Design review of the part built by this model. Coordinates are the model's own, in mm. A direction names the side the tool comes from. Give positions to 0.01 mm unless a question says otherwise; leave off trailing zeros. Loops run counter-clockwise (first coordinate to the right, second up) from the corner with the lowest first, then second, coordinate; pieces in that order, holes last. Notation, with made-up numbers: M 7.25,-28.75 L 37.25,-28.75 A17 cw 37.25,-0.75 Z; hole C -10.5,86.5 d3. An arc over 180 degrees is marked long. Answer as CSV lines item,"result".
```python
from build123d import *

# Parameters (mm, degrees)
F0_W     = 60
F0_H     = 200
F1_DEPTH = 10
F2_W     = 30
F2_H     = 20
F3_DEPTH = 30
F4_W     = 50
F4_H     = 152
F5_DEPTH = 8
F6_R     = 12.472601
F7_DEPTH = 60.001


with BuildPart() as f1:
    # F0 (on Top) → F1 (new body)
    with BuildSketch(Plane.XY):
        Rectangle(F0_W, F0_H)
    extrude(amount=F1_DEPTH)

    # F2 (on Right) → F3 (join, symmetric)
    with BuildSketch(Plane.YZ):
        with Locations((-85, -10)):
            Rectangle(F2_W, F2_H)
        with Locations((85, -10)):
            Rectangle(F2_W, F2_H)
    extrude(amount=F3_DEPTH, both=True)

    # F4 (on face) → F5 (join)
    with BuildSketch(Plane.XY.offset(10)):
        Rectangle(F4_W, F4_H)
    extrude(amount=F5_DEPTH)

    # F6 (on face) → F7 (cut, through all)
    with BuildSketch(Plane.YZ.offset(30)):
        with Locations((-85, -5)):
            Circle(F6_R)
        with Locations((85, -5)):
            Circle(F6_R)
    extrude(amount=-F7_DEPTH, mode=Mode.SUBTRACT)


solid = f1.part
```
1. For faces 1 (the flat face through (0, -70, -10)), 2 (the flat face through (25, -1, 14)), 3 (the flat face through (0, -76, 14)), list the 3-axis set-ups (+Z, -Z, +X, -X, +Y, -Y) from which the entire face can be reached by the end or side of a thin tool; tool diameter is ignored.
Answer block:
face 1,"-Z, +X, -X"
face 2,"+Z, +X, +Y, -Y"
face 3,"+Z, +X, -X, -Y"
2. We need section A-A, the plane y = -85. Write out the cut boundary in (x, z), plus the area to 3 significant figures.
Answer block:
outline,"M -30,-20 L 30,-20 L 30,-17.47 L -30,-17.47 Z; M -30,7.47 L 30,7.47 L 30,10 L -30,10 Z"
area,"303 mm²"
3. We need section B-B, the plane z = -5. Write out the cut boundary in (x, y).
Answer block:
outline,"M -30,-100 L 30,-100 L 30,-97.47 L -30,-97.47 Z; M -30,-72.53 L 30,-72.53 L 30,-70 L -30,-70 Z; M -30,70 L 30,70 L 30,72.53 L -30,72.53 Z; M -30,97.47 L 30,97.47 L 30,100 L -30,100 Z"
4. We need section D-D, the plane y = -41.5. Write out the cut boundary in (x, z), plus the area to 3 significant figures.
Answer block:
outline,"M -30,0 L 30,0 L 30,10 L 25,10 L 25,18 L -25,18 L -25,10 L -30,10 Z"
area,"1,000 mm²"
5. To check wall thickness, follow L1, parallel to Z at x = 7, y = -85; L2, parallel to Y at x = -15.5, z = 0.5; L3, parallel to Y at x = -24.5, z = 6. State the ranges of each line that lie inside material, in increasing order. Write a range as [from, to].
Answer block:
L1,"[-20, -17.47], [7.47, 10]"
L2,"[-100, -96.19], [-73.81, 73.81], [96.19, 100]"
L3,"[-100, -90.88], [-79.12, 79.12], [90.88, 100]"
6. For P1, Ø4, axis at x = 8.5, z = 15.5, coming from the -Y side; P2, Ø6.5, axis at y = -5, z = 14, coming from the +X side; P3, Ø6, axis at x = -8, y = 66, coming from the -Z side; P4, Ø22.5, axis at y = -85, z = -5, coming from the +X side, all flat-tipped, find the tip position at first contact; note any pin that passes through.
Answer block:
P1,"y = -76"
P2,"x = 25"
P3,"z = 0"
P4,"through"
7. We need section C-C, the plane z = 4. Write out the cut boundary in (x, y), plus the area to 3 significant figures.
Answer block:
outline,"M -30,-100 L 30,-100 L 30,-93.64 L -30,-93.64 Z; M -30,-76.36 L 30,-76.36 L 30,76.36 L -30,76.36 Z; M -30,93.64 L 30,93.64 L 30,100 L -30,100 Z"
area,"9,930 mm²"
